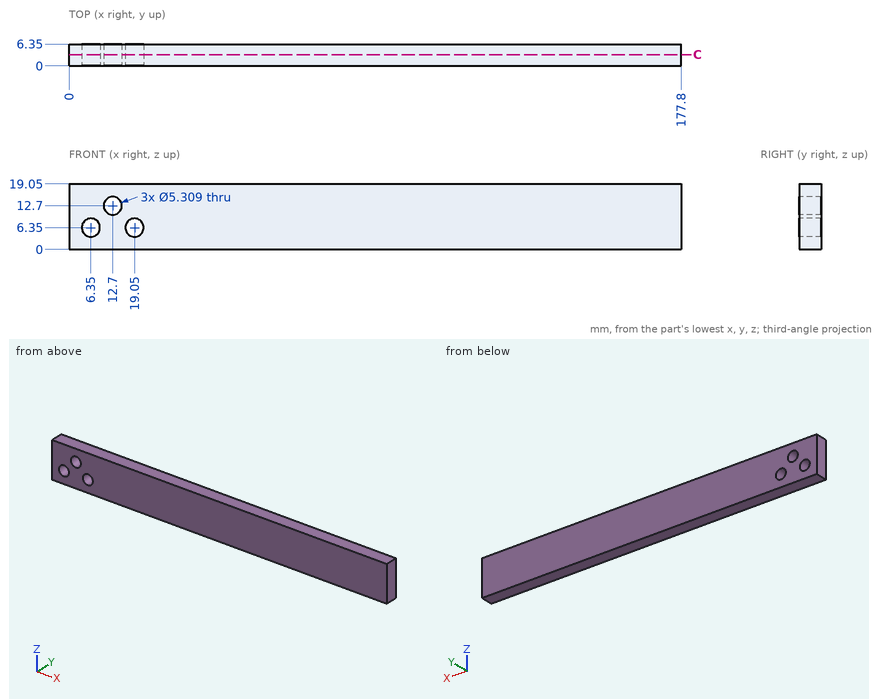
Geometry check sheet. Reference: drawing and pictorial views, mm from the part's lowest x, y, z. Coordinates: 2 decimals unless noted, no trailing zeros. Return JSON: item names as keys, results as strings.
1) Thickness scan on L1, parallel to X at y = 4, z = 6.35 (1 decimal); L2, parallel to X at y = 6, z = 5.25 (1 decimal); L3, parallel to X at y = 5.75, z = 13. Record the ranges inside material, lowest first. Write a range as [from, to].
Answer list:
{"L1": "[0, 3.7], [9, 16.4], [21.7, 177.8]", "L2": "[0, 3.9], [8.8, 16.6], [21.5, 177.8]", "L3": "[0, 10.06], [15.34, 177.8]"}
2) Cross-section at C-C, the plane y = 3.25. Count the separate pieces of the cut face and the enclosed holes in it, and give its area (3 significant figures).
Answer list:
{"separate pieces": "1", "enclosed holes": "3", "area": "3,320 mm2"}
3) Gauge pin test, flat end, axial feed: pin 1 (5 mm diameter, centred on x = 19.05, z = 6.35, fed in from +Y). Record the tip position at first contact, or that the pin passes through.
Answer list:
{"pin 1": "through"}
